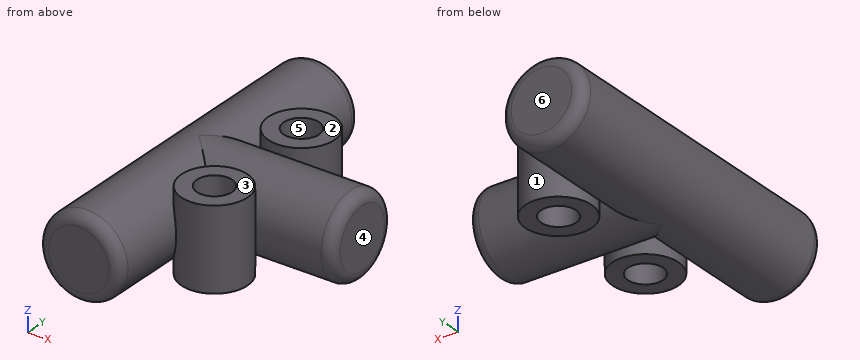
Autodesk Inventor part; units mm, degrees
ref_plane "YZ Plane" through (0, 0, 0) normal (1, 0, 0) x (0, 1, 0)
ref_plane "XZ Plane" through (0, 0, 0) normal (0, 1, 0) x (-1, 0, 0)
ref_plane "XY Plane" through (0, 0, 0) normal (0, 0, 1) x (1, 0, 0)
sketch "Sketch1" plane through (0, 0, 0) normal (0, 1, 0) x (-1, 0, 0)
  circle A0 centre (0, 0) radius 3.75
  dimension "d0" = 7.5
extrude "Extrusion1" add sketch "Sketch1" along normal mid plane 29.8
sketch "Sketch2" plane through (0, 0, 0) normal (1, 0, 0) x (0, 1, 0)
  line L0 (-14.9, 3.75) -> (-14.9, -3.75)
  line L1 (14.9, -3.75) -> (14.9, 3.75)
  circle A0 centre (0, 0) radius 3.75
extrude "Extrusion2" add sketch "Sketch2" along normal blind 14.9
sketch "Sketch3" plane through (0, 0, 0) normal (0, 0, 1) x (1, 0, 0)
  line L0 (0, 13.8301) -> (0, -13.8301) construction
  line L1 (-5.2476, 0) -> (14.0163, 0) construction
  circle A0 centre (5.4, 5.4) radius 1.6
  circle A1 centre (5.4, -5.4) radius 1.6
  circle A2 centre (5.4, 5.4) radius 3
  circle A3 centre (5.4, -5.4) radius 3
  point P0 (0, 0)
  point P1 (0, 0)
  dimension "d5" = 5.4
  dimension "d6" = 5.4
  dimension "d7" = 3.2
  dimension "d8" = 3.2
  dimension "d9" = 6
  dimension "d10" = 6
  dimension "d11" = 5.4
  dimension "d12" = 5.4
extrude "Extrusion3" add sketch "Sketch3" along normal mid plane 7.4
fillet "Fillet1" radius 1 3 edges at (3.75, 14.9, 0) (14.9, -3.75, 0) (3.75, -14.9, 0)
properties part number "Union Tee 1-8 KQ2T01-00A SMC"
CAD build for the part. Positions are in the model's coordinates, mm. Face numbers are marked on the shaded views. A direction names the side the tool comes from. Coordinates: 2 decimals unless noted, no trailing zeros. Loops run counter-clockwise (first coordinate to the right, second up) from the corner with the lowest first, then second, coordinate; pieces in that order, holes last. Notation, with made-up numbers: (88, 24) - (147, 24) arc R11 cw to (147, 34) - close; hole circle Ø6 at (29, 14). An arc over 180 degrees is marked (long way). Use CSV: the item, a comma, the result in double quotes. Start each with the question number.
Q1. Two-plate mould, pull along X, no slides. Class the marked faces 4, 5 and 6: +X half, -X half, draft (parallel to the pull), parting line (faces both ways), or undercut.
Q2. Drop flat-ended pins along their axis: P1, Ø6.5, axis at x = 5, y = -4, coming from the -Z side; P2, Ø4, axis at x = 11.5, z = 1, coming from the -Y side; P3, Ø10, axis at x = 7, y = -6.5, coming from the +Z side. Give the stop position or say it passes through.
Q3. Cut at B-B, the plane x = 5.4. List the corners of the cut face in (y, z).
Q4. Cut at C-C, the plane z = 0. List the corners of the cut face in (x, y), then the cut area to 3 significant figures.
Q5. Probe probe 1 along Y at (x, z) = (5.4, 0.75); probe 2 along Y at (x, z) = (4, -2.25); probe 3 along Y at (x, z) = (10, 0). List the from-to ranges inside material, lowest first. Write a range as from..to.
Q6. 3-axis set-ups, long thin cutter, end or side, ignore diameter. For the marked faces 1, 2 and 3: which of +Z, -Z, +X, -X, +Y, -Y reach the whole face in a straight line?
Q7. Cut at A-A, the plane y = 5.4. List the corners of the cut face in (x, z), then the cut area to 3 significant figures.
Here are the results:
1,face 4,"+X half"
1,face 5,"undercut"
1,face 6,"draft"
2,P1,"z = -3.7"
2,P2,"y = -3.75"
2,P3,"z = 3.7"
3,outline,"(-8.4, -3.7) - (-7, -3.7) - (-7, 3.7) - (-8.4, 3.7) - close; (-3.8, -3.7) - (-2.4, -3.7) - (-2.4, -2.88) arc R3.75 ccw to (2.4, -2.88) - (2.4, -3.7) - (3.8, -3.7) - (3.8, 3.7) - (2.4, 3.7) - (2.4, 2.88) arc R3.75 ccw to (-2.4, 2.88) - (-2.4, 3.7) - (-3.8, 3.7) - close; (7, -3.7) - (8.4, -3.7) - (8.4, 3.7) - (7, 3.7) - close"
4,outline,"(-3.75, -13.9) arc R1 ccw to (-2.75, -14.9) - (2.75, -14.9) arc R1 ccw to (3.75, -13.9) - (3.75, -7.91) arc R3 ccw to (7.91, -3.75) - (13.9, -3.75) arc R1 ccw to (14.9, -2.75) - (14.9, 2.75) arc R1 ccw to (13.9, 3.75) - (7.91, 3.75) arc R3 ccw to (3.75, 7.91) - (3.75, 13.9) arc R1 ccw to (2.75, 14.9) - (-2.75, 14.9) arc R1 ccw to (-3.75, 13.9) - close; hole circle Ø3.2 at (5.4, -5.4); hole circle Ø3.2 at (5.4, 5.4)"
4,area,"328 mm2"
5,probe 1,"-8.4..-7, -3.8..3.8, 7..8.4"
5,probe 2,"-8.05..-6.17, -4.63..4.63, 6.17..8.05"
5,probe 3,"-3.75..3.75"
6,face 1,"none"
6,face 2,"+Z, +X, +Y"
6,face 3,"+Z, +X, -Y"
7,outline,"(2.4, -3.7) - (3.8, -3.7) - (3.8, 3.7) - (2.4, 3.7) - (2.4, 2.88) arc R3.75 ccw (long way) to (2.4, -2.88) - close; (7, -3.7) - (8.4, -3.7) - (8.4, 3.7) - (7, 3.7) - close"
7,area,"59.5 mm2"
